Source: CAD feature listing. Evaluate the final solid. Frame: model axes, mm. A direction names the side the tool comes from. Round coordinates to 2 decimals unless told otherwise and drop trailing zeros. Order: outer loops, then holes, each group sorted by start corner. A loop starts at its lowest first (then second) coordinate and runs counter-clockwise, first axis right, second up. Notation, with made-up numbers: M -8,-35 L -1,-35 A16 cw -1,-27 Z; hole C 40.5,17 d11. An arc over 180 degrees is marked long. Answer as CSV lines item,"result". Start each with the question number.
Item 1: Line query: line 1 (X direction, y = 1.5, z = 14); line 2 (Z direction, x = -20.5, y = 0); line 3 (X direction, y = 10, z = 46). Output: solid intervals per line, ascending. Write a range as [from, to].
Item 2: Pull-direction query (X, two-part tool) for faces 1 (the face through (7, 2, 99)), 2 (the face through (10, 0, 99)), 3 (the face through (-7, 0, 48)), 4 (the face through (14, 0, 105)); classes: +X half, -X half, draft (parallel to the pull), parting line (faces both ways), or undercut.
Item 3: First-contact query: P1, Ø0.6, axis at x = -5.5, z = 47.5, coming from the +Y side; P2, Ø0.6, axis at x = 13, y = -8.5, coming from the -Z side; P3, Ø3, axis at x = 3, y = 0, coming from the -Z side; P4, Ø1, axis at y = -9.5, z = 97, coming from the +X side. Flat tips, straight axial feed; report the tip coordinate or a pass-through.
Item 4: Set-up query: faces 5 (the face through (5, 0, 100)), 6 (the face through (2, -2, 22)), 7 (the face through (-16, 0, 25)). Return all of +Z, -Z, +X, -X, +Y, -Y with unobstructed straight access to the full face (end or side cutting, diameter ignored); none if empty.
Item 5: Section query C-C on x = 1.5. Return the cut outline in (y, z), plus the area to 3 significant figures.
Item 6: Section query B-B on z = 44. Return the cut outline in (x, y).
Item 7: Section query D-D on z = 100.5. Return the cut outline in (x, y).
Item 8: Section query A-A on y = 3.5. Return the cut outline in (x, z).
Autodesk Fusion 360 part; units mm, degrees
sketch "스케치1" plane through (0, 0, 0) normal (0, 1, 0) x (1, 0, 0)
  line L0 (-25, 0) -> (-25, -25)
  line L1 (-25, -25) -> (25, -25)
  line L2 (25, -25) -> (25, 0)
  line L3 (25, 0) -> (21, 0)
  line L4 (21, 0) -> (21, -21)
  line L5 (21, -21) -> (-21, -21)
  line L6 (-21, -21) -> (-21, 0)
  line L7 (-21, 0) -> (-25, 0)
extrude "돌출1" add sketch "스케치1" along normal mid plane 4
sketch "스케치2" plane through (0, 0, 25) normal (0, 0, 1) x (-1, 0, 0)
  line L0 (25, 2) -> (-25, 2)
  line L1 (5, -13) -> (-5, -13)
  line L2 (5, -13) -> (5, 0)
  line L3 (-5, -13) -> (-5, 0)
  line L4 (-20, 0) -> (-2.5, 0)
  line L5 (5, 13) -> (-5, 13)
  line L6 (5, 13) -> (5, 0)
  line L7 (-5, 13) -> (-5, 0)
extrude "돌출2" add sketch "스케치2" along normal blind 70
sketch "스케치4" plane through (5, 0, 0) normal (1, 0, 0) x (0, 1, 0)
  line L0 (7.5, 25) -> (-7.5, 25)
  line L1 (-7.5, 25) -> (-7.5, 67.4494)
  line L2 (-7.5, 67.4494) -> (7.5, 67.4494)
  line L3 (7.5, 67.4494) -> (7.5, 25)
  line L4 (2, 25) -> (13, 25)
extrude "돌출3" add sketch "스케치4" along normal blind 7
sketch "스케치5" plane through (-5, 0, 0) normal (-1, 0, 0) x (0, -1, 0)
  line L0 (-10.25, 25) -> (10, 25)
  line L1 (10, 25) -> (10, 70)
  line L2 (10, 70) -> (-10.25, 70)
  line L3 (-10.25, 70) -> (-10.25, 25)
  line L4 (-7.5, 25) -> (-13, 25)
extrude "돌출4" add sketch "스케치5" along normal blind 2
sketch "스케치7" plane through (-5, 0, 0) normal (-1, 0, 0) x (0, -1, 0)
  line L0 (-12, 72) -> (12, 72)
  line L1 (12, 72) -> (12, 93)
  line L2 (12, 93) -> (-12, 93)
  line L3 (-12, 93) -> (-12, 72)
extrude "돌출5" add sketch "스케치7" along normal blind 20
sketch "스케치10" plane through (5, 0, 0) normal (1, 0, 0) x (0, 1, 0)
  line L0 (-2, 93) -> (2, 93)
  line L1 (2, 93) -> (2, 105)
  line L2 (2, 105) -> (-2, 105)
  line L3 (-2, 105) -> (-2, 93)
  line L4 (-12, 93) -> (12, 93)
extrude "돌출7" add sketch "스케치10" along normal blind 5
sketch "스케치12" plane through (10, 0, 0) normal (1, 0, 0) x (0, 1, 0)
  circle A0 centre (0, 103.5) radius 0.5
extrude "돌출8" add sketch "스케치12" along normal blind 4
sketch "스케치13" plane through (14, 0, 0) normal (1, 0, 0) x (0, 1, 0)
  circle A0 centre (0, 103.5) radius 18.5
  circle A1 centre (0, 103.5) radius 0.5
  line L0 (-0.5, 104) -> (-0.5, 120.9929)
  line L1 (0.5, 104) -> (0.5, 120.9929)
  line L2 (-0.5, 103) -> (-17.4929, 103)
  line L3 (-0.5, 104) -> (-17.4929, 104)
  line L4 (0.5, 103) -> (0.5, 86.0071)
  line L5 (-0.5, 103) -> (-0.5, 86.0071)
  line L6 (0.5, 104) -> (17.4929, 104)
  line L7 (0.5, 103) -> (17.4929, 103)
  arc A2 (-0.5, 103.5) -> (0, 103) centre (0, 103.5) ccw
  arc A3 (-0.5, 120.9929) -> (-17.4929, 104) centre (0, 103.5) ccw
  arc A4 (17.4929, 104) -> (0.5, 120.9929) centre (0, 103.5) ccw
  arc A5 (-17.4929, 103) -> (-0.5, 86.0071) centre (0, 103.5) ccw
  arc A6 (0.5, 86.0071) -> (17.4929, 103) centre (0, 103.5) ccw
  point P0 (-0.5, 103.5)
  dimension "d23" = 17.5
  dimension "d24" = 37
extrude "돌출9" add sketch "스케치13" against normal blind 2
Results:
1,line 1,"[-25, -21], [21, 25]"
1,line 2,"[21, 25], [72, 93]"
1,line 3,"[-7, 5]"
2,face 1,"draft"
2,face 2,"undercut"
2,face 3,"-X half"
2,face 4,"+X half"
3,P1,"y = 10.25"
3,P2,"z = 86.92"
3,P3,"z = 21"
3,P4,"through"
4,face 5,"+Z, -X, +Y, -Y"
4,face 6,"-Z, +X, -X, -Y"
4,face 7,"-X, +Y, -Y"
5,outline,"M -13,25 L -2,25 L -2,21 L 2,21 L 2,25 L 13,25 L 13,95 L -13,95 Z"
5,area,"1,840 mm^2"
6,outline,"M -7,-10 L -5,-10 L -5,-13 L 5,-13 L 5,-7.5 L 12,-7.5 L 12,7.5 L 5,7.5 L 5,13 L -5,13 L -5,10.25 L -7,10.25 Z"
7,outline,"M 5,-2 L 10,-2 L 10,2 L 5,2 Z; M 12,-18.26 L 14,-18.26 L 14,-17.24 L 12,-17.24 Z; M 12,-0.5 L 14,-0.5 L 14,0.5 L 12,0.5 Z; M 12,17.24 L 14,17.24 L 14,18.26 L 12,18.26 Z"
8,outline,"M -25,72 L -5,72 L -5,70 L -7,70 L -7,25 L 12,25 L 12,67.45 L 5,67.45 L 5,95 L -5,95 L -5,93 L -25,93 Z; M 12,85.33 L 14,85.33 L 14,86.35 L 12,86.35 Z; M 12,103 L 14,103 L 14,104 L 12,104 Z; M 12,120.65 L 14,120.65 L 14,121.67 L 12,121.67 Z"
